Geometry: final body of the model. Coordinates: model frame, mm. Face numbers are marked on the shaded views. A direction names the side the tool comes from. Give positions to 0.01 mm unless a question says otherwise; leave off trailing zeros. Write each loop counter-clockwise with the first axis right and the second up, starting at its lowest first coordinate (ties: lowest second). Pieces come first, ordered by that corner, then holes. Notation, with made-up numbers: M 7.25,83.5 L 33.25,83.5 A14 ccw 33.25,107.5 Z; hole C 3.25,28.5 d7. An arc over 180 degrees is marked long. Use a Markdown table: item, result. Add a question column.
1) Set-up query: the marked faces 5 and 6. Return all of +Z, -Z, +X, -X, +Y, -Y with unobstructed straight access to the full face (end or side cutting, diameter ignored); none if empty.
2) Draft query along X for the marked faces 1, 2, 3 and 4. Return one class per face: +X half, -X half, draft (parallel to the pull), parting line (faces both ways), or undercut.
3) Section C-C on z = 48.5. Return the cut outline in (x, y).
4) Section D-D on x = 18.5. Return the cut outline in (y, z).
5) Line query: line 1 (Y direction, x = -0.5, z = 11.5); line 2 (X direction, y = -31, z = 9); line 3 (Z direction, x = 18.5, y = -26.5). Output: solid intervals per line, ascending.
6) Section B-B on x = -39. Return the cut outline in (y, z), then the cut area to 3 significant figures.
7) Pin query (flat end, axial travel): pin 1 (2 mm diameter, centred on y = -9.5, z = 10, fed in from +X); pin 2 (6 mm diameter, centred on x = 7, y = -27, fed in from +Z); pin 3 (1.5 mm diameter, centred on y = -7.5, z = 19, fed in from +X). Return the tip coordinate at first contact, or that it passes through.
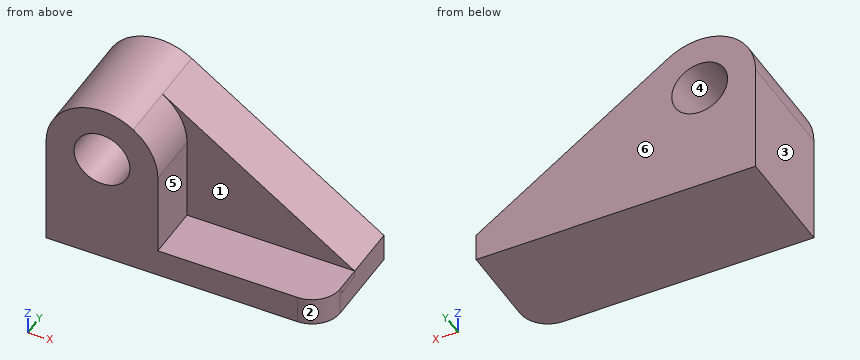
```python
from build123d import *

# Parameters (mm, degrees)
F0_R        = 12.7
F1_DEPTH    = 25.4
F2_R        = 12.7
F3_DEPTH    = 25.4
F4_T1_DEPTH = 73.3820900713
F4_T6_DEPTH = 61.9223878104


# Not quite as in the source:
# - a fillet or chamfer that OpenCascade refuses, or shapes differently, is made with other operations: its cross-section is extruded or revolved along the edge and cut away or added


with BuildPart() as f1:
    # F0 (on Front) → F1 (new body)
    with BuildSketch(Plane.XZ):
        with BuildLine():
            Line((51.8036965728, 2.8171599331), (-35.5584302991, 61.9514882749))
            ThreePointArc((-35.5584302991, 61.9514882749), (-61.7025627589, 63.353759246), (-75.1963034272, 40.9171599331))
            Line((-75.1963034272, 40.9171599331), (-75.1963034272, -9.8828400669))
            Line((-75.1963034272, -9.8828400669), (51.8036965728, -9.8828400669))
            Line((51.8036965728, -9.8828400669), (51.8036965728, 2.8171599331))
        make_face()
        with Locations((-49.7963034272, 40.9171599331)):
            Circle(F0_R, mode=Mode.SUBTRACT)
    extrude(amount=F1_DEPTH)

    # F2 (on face) → F3 (join)
    with BuildSketch(Plane.XZ.offset(25.4)):
        with BuildLine():
            Line((-24.3963034272, 2.8171599331), (-24.3963034272, 40.9171599331))
            ThreePointArc((-24.3963034272, 40.9171599331), (-27.3597041143, 52.8234192648), (-35.5584302991, 61.9514882749))
            ThreePointArc((-35.5584302991, 61.9514882749), (-61.7025627589, 63.353759246), (-75.1963034272, 40.9171599331))
            Line((-75.1963034272, 40.9171599331), (-75.1963034272, 0))
            Line((-75.1963034272, 0), (-75.1963034272, -9.8828400669))
            Line((-75.1963034272, -9.8828400669), (51.8036965728, -9.8828400669))
            Line((51.8036965728, -9.8828400669), (51.8036965728, -0.3670600709))
            Line((51.8036965728, -0.3670600709), (51.8036965728, 0))
            Line((51.8036965728, 0), (51.7987225249, 0))
            Line((51.7987225249, 0), (51.8036965728, 2.8171599331))
            Line((51.8036965728, 2.8171599331), (-24.3963034272, 2.8171599331))
        make_face()
        with Locations((-49.7963034272, 40.9171599331)):
            Circle(F2_R, mode=Mode.SUBTRACT)
    extrude(amount=F3_DEPTH)

    # F4: fillet of radius 12.7 on 2 edges, made by hand

    # F4_s2 → F4_t1 (cut)
    with BuildSketch(Plane.XY.offset(-41.6324650691)):
        with BuildLine():
            ThreePointArc((39.1038465728, -50.80015), (48.0841026938, -47.0804061211), (51.8038465728, -38.10015))
            Line((51.8038465728, -38.10015), (52.0578465728, -38.10015))
            ThreePointArc((52.0578465728, -38.10015), (52.0576965728, -44.450075), (52.0576965728, -50.8))
            Line((52.0576965728, -50.8), (51.8036965728, -51.054))
            ThreePointArc((51.8036965728, -51.054), (45.4537715728, -51.054), (39.1038465728, -51.05415))
            Line((39.1038465728, -51.05415), (39.1038465728, -50.80015))
        make_face()
    extrude(amount=F4_T1_DEPTH, mode=Mode.SUBTRACT)


with BuildPart() as f4_tool4:
    # F4_s5 → F4_t6 (new body)
    with BuildSketch(Plane.YZ.offset(82.762403454)):
        with BuildLine():
            ThreePointArc((-50.8001462633, -9.8828067947), (-46.3384346707, -2.7734597017), (-38.4165172484, 0.00015))
            Line((-38.4165172484, 0.00015), (-38.4165172484, 0.25415))
            ThreePointArc((-38.4165172484, 0.25415), (-44.6082586242, 0.254), (-50.8, 0.254))
            Line((-50.8, 0.254), (-51.054, 0))
            ThreePointArc((-51.054, 0), (-51.054, -4.9414033973), (-51.0478188436, -9.8264659306))
            Line((-51.0478188436, -9.8264659306), (-50.8001462633, -9.8828067947))
        make_face()
    extrude(amount=-F4_T6_DEPTH)

    split(bisect_by=Plane(origin=(51.7985610464, 0, -0.0914568329), x_dir=(0, 1, 0), z_dir=(0.9999984413, 0, -0.0017656222)), keep=Keep.TOP)


with BuildPart() as f1_1:
    add(f1.part)

    # F4_t3: cut F4_tool4
    add(f4_tool4.part, mode=Mode.SUBTRACT)


solid = f1_1.part
```
Found:
| question | item | result |
|---|---|---|
| 1 | face 5 | +Z, +X, -Y |
| 1 | face 6 | +Z, -Z, +X, -X, +Y |
| 2 | face 1 | draft |
| 2 | face 2 | +X half |
| 2 | face 3 | -X half |
| 2 | face 4 | undercut |
| 3 | outline | M -74.04,-50.8 L -59.98,-50.8 L -59.98,0 L -74.04,0 Z; M -39.61,-50.8 L -25.55,-50.8 L -25.55,-25.4 L -15.69,-25.4 L -15.69,0 L -39.61,0 Z |
| 4 | outline | M -50.8,-9.88 L 0,-9.88 L 0,25.36 L -25.4,25.36 L -25.4,2.82 L -50.8,2.82 Z |
| 5 | line 1 | -25.4 to 0 |
| 5 | line 2 | -75.2 to -24.4 |
| 5 | line 3 | -9.88 to 2.82 |
| 6 | outline | M -50.8,-9.88 L 0,-9.88 L 0,34.23 L -50.8,34.23 Z; M -50.8,47.61 L 0,47.61 L 0,63.91 L -50.8,63.91 Z |
| 6 | area | 3,070 mm² |
| 7 | pin 1 | x = 42.67 |
| 7 | pin 2 | z = 34.86 |
| 7 | pin 3 | x = 29 |
